from build123d import *

# Parameters (mm, degrees)
FILLET1_R                  = 0.7874
SKETCH2_W                  = 4.4831
SKETCH2_H                  = 32.8676
CUT_EXTRUDE1_DEPTH         = 12.1125
CUT_EXTRUDE1_DEPTH_BACK    = 12.1125
SKETCH3_R                  = 5.9944
SKETCH3_R_2                = 4.8895
CUT_EXTRUDE2_DEPTH         = 2.54
CHAMFER1_SIZE              = 0.762
SKETCH4_R                  = 5.55879
EXTRUDE1_DEPTH             = 15.875
CHAMFER2_SIZE              = 0.381
CHAMFER2_SIZE2             = 2.160758373
FILLET2_R                  = 2.286
EXTRUDE2_DEPTH             = 7.5057
EXTRUDE2_DEPTH_BACK        = 7.5057
CUT_EXTRUDE3_START         = 5.588
SKETCH6_R                  = 5.2451
CUT_EXTRUDE3_DEPTH         = 15.6558
SKETCH7_R                  = 5.0038
EXTRUDE3_DEPTH             = 5.9944
CHAMFER3_SIZE              = 0.762
CUT_EXTRUDE4_DEPTH         = 5.0038
EXTRUDE4_REACH             = 23.006
SKETCH10_R                 = 2.9972
EXTRUDE4_DIRECTION_2_REACH = 23.006
SKETCH11_R                 = 20.6375
SKETCH11_R_2               = 11.1125
EXTRUDE5_DEPTH             = 6.35


with BuildPart() as part:
    # Sketch1 → Revolve1 (revolve)
    with BuildSketch(Plane(origin=(0, 0, 0), x_dir=(0, 0, -1), z_dir=(1, 0, 0))):
        Polygon((0, 41.656), (11.1125, 41.656), (11.1125, 1.1684), (5.9944, 1.1684), (5.9944, -11.5316), (0, -11.5316), align=None)
    revolve(axis=Axis((0, -15.35938, 0), (0, 1, 0)))

    # Fillet1
    fillet1_edges = [part.edges().sort_by_distance(p)[0] for p in [
        (0, 41.656, 11.1125),
    ]]
    fillet(fillet1_edges, radius=FILLET1_R)

    # Sketch2 → Cut-Extrude1 (cut, two sides)
    with BuildSketch(Plane.XY) as cut_extrude1_sk:
        with Locations((8.87095, 25.2222)):
            Rectangle(SKETCH2_W, SKETCH2_H)
        with Locations((-8.87095, 25.2222)):
            Rectangle(SKETCH2_W, SKETCH2_H)
    extrude(amount=CUT_EXTRUDE1_DEPTH, mode=Mode.SUBTRACT)
    extrude(cut_extrude1_sk.sketch, amount=-CUT_EXTRUDE1_DEPTH_BACK, mode=Mode.SUBTRACT)

    # Sketch3 → Cut-Extrude2 (cut)
    with BuildSketch(Plane.XZ.offset(-1.1684)):
        with Locations(Location((0, 0, 0), (0, 0, 270))):  # turned: the seam where the file's is
            Circle(SKETCH3_R)
        with Locations(Location((0, 0, 0), (0, 0, 270))):  # turned: the seam where the file's is
            Circle(SKETCH3_R_2, mode=Mode.SUBTRACT)
    extrude(amount=CUT_EXTRUDE2_DEPTH, mode=Mode.SUBTRACT)

    # Chamfer1
    chamfer1_edges = [part.edges().sort_by_distance(p)[0] for p in [
        (0, -11.5316, 5.9944),
    ]]
    chamfer(chamfer1_edges, length=CHAMFER1_SIZE)

    # Sketch4 → Extrude1 (add, symmetric)
    with BuildSketch(Plane(origin=(0, 0, 0), x_dir=(0, 0, -1), z_dir=(1, 0, 0))):
        with Locations(Location((0, 27.7876, 0), (0, 0, 90))):  # turned: the seam where the file's is
            Circle(SKETCH4_R)
    extrude(amount=EXTRUDE1_DEPTH, both=True)

    # Chamfer2
    chamfer2_edges = [part.edges().sort_by_distance(p)[0] for p in [
        (15.875, 22.22881, 0),
    ]]
    chamfer2_side = [part.faces().sort_by_distance(p)[0] for p in [
        (15.875, 27.7876, 0),
    ]]
    chamfer(chamfer2_edges, length=CHAMFER2_SIZE, length2=CHAMFER2_SIZE2, reference=chamfer2_side[0])

    # Fillet2
    fillet2_edges = [part.edges().sort_by_distance(p)[0] for p in [
        (-15.875, 22.22881, 0),
    ]]
    fillet(fillet2_edges, radius=FILLET2_R)

    # Sketch5 → Extrude2 (add, two sides)
    with BuildSketch(Plane(origin=(0, 0, 0), x_dir=(1, 0, 0), z_dir=(0, 1, 0))) as extrude2_sk:
        with BuildLine():
            Line((11.086343502, 0.762), (20.99197441, 0.762))
            ThreePointArc((20.99197441, 0.762), (0, 21.0058), (-20.99197441, 0.762))
            Line((-20.99197441, 0.762), (-11.086343502, 0.762))
            ThreePointArc((-11.086343502, 0.762), (0, 11.1125), (11.086343502, 0.762))
        make_face()
        with BuildLine():
            Line((11.086343502, -0.762), (20.99197441, -0.762))
            ThreePointArc((20.99197441, -0.762), (0, -21.0058), (-20.99197441, -0.762))
            Line((-20.99197441, -0.762), (-11.086343502, -0.762))
            ThreePointArc((-11.086343502, -0.762), (0, -11.1125), (11.086343502, -0.762))
        make_face()
    extrude(amount=EXTRUDE2_DEPTH)
    extrude(extrude2_sk.sketch, amount=-EXTRUDE2_DEPTH_BACK)

    # Sketch6 → Cut-Extrude3 (cut, through all)
    with BuildSketch(Plane.XY.offset(0.762).offset(CUT_EXTRUDE3_START)):
        with Locations((15.875, 0)):
            Circle(SKETCH6_R)
        with Locations((-15.875, 0)):
            Circle(SKETCH6_R)
    extrude(amount=CUT_EXTRUDE3_DEPTH, mode=Mode.SUBTRACT)

    # Sketch7 → Extrude3 (add)
    with BuildSketch(Plane.XY.offset(6.35)):
        with Locations(Location((15.875, 0, 0), (0, 0, 325.993384386))):  # turned: the seam where the file's is
            Circle(SKETCH7_R)
        with Locations(Location((-15.875, 0, 0), (0, 0, 214.006615614))):  # turned: the seam where the file's is
            Circle(SKETCH7_R)
    extrude(amount=EXTRUDE3_DEPTH)

    # Chamfer3
    chamfer3_edges = [part.edges().sort_by_distance(p)[0] for p in [
        (11.726984901, 2.798568416, 12.3444),
        (-11.726984901, 2.798568416, 12.3444),
    ]]
    chamfer(chamfer3_edges, length=CHAMFER3_SIZE)

    # Sketch8 → Cut-Extrude4 (cut)
    with BuildSketch(Plane.XY.offset(12.3444)):
        Polygon((17.319472638, 2.5019), (18.763945277, 0), (17.319472638, -2.5019), (14.430527362, -2.5019), (12.986054723, 0), (14.430527362, 2.5019), align=None)
        Polygon((-18.763945277, 0), (-17.319472638, -2.5019), (-14.430527362, -2.5019), (-12.986054723, 0), (-14.430527362, 2.5019), (-17.319472638, 2.5019), align=None)
    extrude(amount=-CUT_EXTRUDE4_DEPTH, mode=Mode.SUBTRACT)

    # Sketch10 → Extrude4 (add, up to next)
    with BuildSketch(Plane.XY, mode=Mode.PRIVATE) as extrude4_sk1:
        with Locations((15.875, 0)):
            Circle(SKETCH10_R)
    extrude4_tool1 = extrude(extrude4_sk1.sketch, amount=EXTRUDE4_REACH, mode=Mode.PRIVATE) - part.part
    add(extrude4_tool1.solids().sort_by_distance((15.875, 0, 0))[0])
    # Sketch10 → Extrude4 (add, up to next)
    with BuildSketch(Plane.XY, mode=Mode.PRIVATE) as extrude4_sk2:
        with Locations((-15.875, 0)):
            Circle(SKETCH10_R)
    extrude4_tool2 = extrude(extrude4_sk2.sketch, amount=EXTRUDE4_REACH, mode=Mode.PRIVATE) - part.part
    add(extrude4_tool2.solids().sort_by_distance((-15.875, 0, 0))[0])

    # Sketch10 → Extrude4 direction 2 (add, up to next)
    with BuildSketch(Plane.XY, mode=Mode.PRIVATE) as extrude4_direction_2_sk1:
        with Locations((15.875, 0)):
            Circle(SKETCH10_R)
    extrude4_direction_2_tool1 = extrude(extrude4_direction_2_sk1.sketch, amount=-EXTRUDE4_DIRECTION_2_REACH, mode=Mode.PRIVATE) - part.part
    add(extrude4_direction_2_tool1.solids().sort_by_distance((15.875, 0, 0))[0])
    # Sketch10 → Extrude4 direction 2 (add, up to next)
    with BuildSketch(Plane.XY, mode=Mode.PRIVATE) as extrude4_direction_2_sk2:
        with Locations((-15.875, 0)):
            Circle(SKETCH10_R)
    extrude4_direction_2_tool2 = extrude(extrude4_direction_2_sk2.sketch, amount=-EXTRUDE4_DIRECTION_2_REACH, mode=Mode.PRIVATE) - part.part
    add(extrude4_direction_2_tool2.solids().sort_by_distance((-15.875, 0, 0))[0])

    # Sketch11 → Extrude5 (add)
    with BuildSketch(Plane(origin=(0, 7.5057, 0), x_dir=(-1, 0, 0), z_dir=(0, 1, 0))):
        with Locations(Location((0, 0, 0), (0, 0, 182.116017459))):  # turned: the seam where the file's is
            Circle(SKETCH11_R)
        Circle(SKETCH11_R_2, mode=Mode.SUBTRACT)
    extrude(amount=EXTRUDE5_DEPTH)


solid = part.part
Input: part model. Units: mm. Frame: model coordinates. A direction names the side the tool comes from. Coordinates: 2 decimals unless noted, no trailing zeros. Order: outer loops, then holes, each group sorted by start corner. A loop starts at its lowest first (then second) coordinate and runs counter-clockwise, first axis right, second up. Notation, with made-up numbers: M 20.25,63.25 L 33.25,63.25 A14 cw 33.25,87.25 Z; hole C -33.75,57.25 d7. An arc over 180 degrees is marked long. One line per question, with ' | ' between items.
Item 1: Section D-D (z = -18). Output: boundary loops of the cut face in (x, y).
Geometry results:
outline: M -10.83,-7.51 L 10.83,-7.51 L 10.83,7.51 L 10.09,7.51 L 10.09,13.86 L -10.09,13.86 L -10.09,7.51 L -10.83,7.51 Z
Item 2: Section B-B (y = 10.5). Output: boundary loops of the cut face in (x, z) (1 decimal).
Geometry results:
outline: C 0,0 d41.3; hole M -6.6,-8.9 L -6.6,8.9 A11.1 ccw Z; hole M 6.6,-8.9 A11.1 ccw 6.6,8.9 Z
Item 3: Section C-C (x = -8). Output: boundary loops of the cut face in (y, z), then the cut area to 3 significant figures.
Geometry results:
outline: M -7.51,-19.42 L 7.51,-19.42 L 7.51,-19.02 L 13.86,-19.02 L 13.86,-7.71 L 8.79,-7.71 L 8.79,7.71 L 13.86,7.71 L 13.86,19.02 L 7.51,19.02 L 7.51,19.42 L -7.51,19.42 L -7.51,7.71 L 1.17,7.71 L 1.17,-7.71 L -7.51,-7.71 Z; C 27.79,0 d11.12 | area: 710 mm^2
Item 4: Pin query (flat end, axial travel): pin 1 (5 mm diameter, centred on x = -18, y = 0, fed in from -Z); pin 2 (10 mm diameter, centred on x = -12, z = 11, fed in from +Y); pin 3 (3 mm diameter, centred on x = 3, y = 15.5, fed in from -Z); pin 4 (5 mm diameter, centred on x = -8, z = 0.5, fed in from +Y). Return the tip coordinate at first contact, or that it passes through.
Geometry results:
pin 1: stops at z = -14.18 | pin 2: stops at y = 13.86 | pin 3: stops at z = -11.01 | pin 4: stops at y = 41.66
Item 5: Draft query along X for faces 4 (the flat face through (15.875, 28, 0)), 5 (the flat face through (16, 7.506, 0)), 6 (the cylindrical face through (10.44, 10.64, -17.8)), 7 (the flat face through (18.052, -1.233, 9.878)). Return one class per face: released by +X, released by -X, zero draft, split by the parting line, or undercut.
Geometry results:
face 4: released by +X | face 5: zero draft | face 6: split by the parting line | face 7: undercut
Item 6: Reachability of faces 1 (the cylindrical face through (10.22, 33.09, 1.67)), 2 (the cylindrical face through (-4.773, -0.084, 1.06)), 3 (the cylindrical face through (-17.708, 4.656, 8.93)) from +Z, -Z, +X, -X, +Y, -Y: full face, straight path, thin tool, end or side. Return the list, or none.
Geometry results:
face 1: +X | face 2: none | face 3: +Z
Item 7: Section A-A (x = 0). Output: boundary loops of the cut face in (y, z).
Geometry results:
outline: M -11.53,-5.23 L -10.77,-5.99 L -1.37,-5.99 L -1.37,-4.89 L 1.17,-4.89 L 1.17,-11.11 L -7.51,-11.11 L -7.51,-21.01 L 7.51,-21.01 L 7.51,-20.64 L 13.86,-20.64 L 13.86,-11.11 L 40.87,-11.11 A0.79 ccw 41.66,-10.33 L 41.66,10.33 A0.79 ccw 40.87,11.11 L 13.86,11.11 L 13.86,20.64 L 7.51,20.64 L 7.51,21.01 L -7.51,21.01 L -7.51,11.11 L 1.17,11.11 L 1.17,4.89 L -1.37,4.89 L -1.37,5.99 L -10.77,5.99 L -11.53,5.23 Z
Item 8: Ray query, line 1 along X through (y, z) = (0, 10); line 2 along Z through (x, y) = (3, -1.5); line 3 along Y through (x, z) = (-11.5, 2). Return the intervals inside material, ascending.
Geometry results:
line 1: x = -20.88 to -18.76, -12.99 to -10.87, -10.63 to -4.85, 4.85 to 10.63, 10.87 to 12.99, 18.76 to 20.88 | line 2: z = -20.79 to -10.7, -5.19 to 5.19, 10.7 to 20.79 | line 3: y = -7.51 to 13.86, 22.6 to 32.97
